For this review, use the dimensioned drawing (mm, ordinates from the lowest corner) and the shaded views. A direction names the side the tool comes from. Give positions to 0.01 mm unless a question says otherwise; leave off trailing zeros. Order: outer loops, then holes, each group sorted by start corner. A loop starts at its lowest first (then second) coordinate and runs counter-clockwise, first axis right, second up. Notation, with made-up numbers: (53, 21) - (62, 21) arc R13 ccw to (62, 37) - close; hole circle Ø4 at (48.25, 59.5). An arc over 180 degrees is marked (long way). Use a Markdown table: item, result. Add a question column.
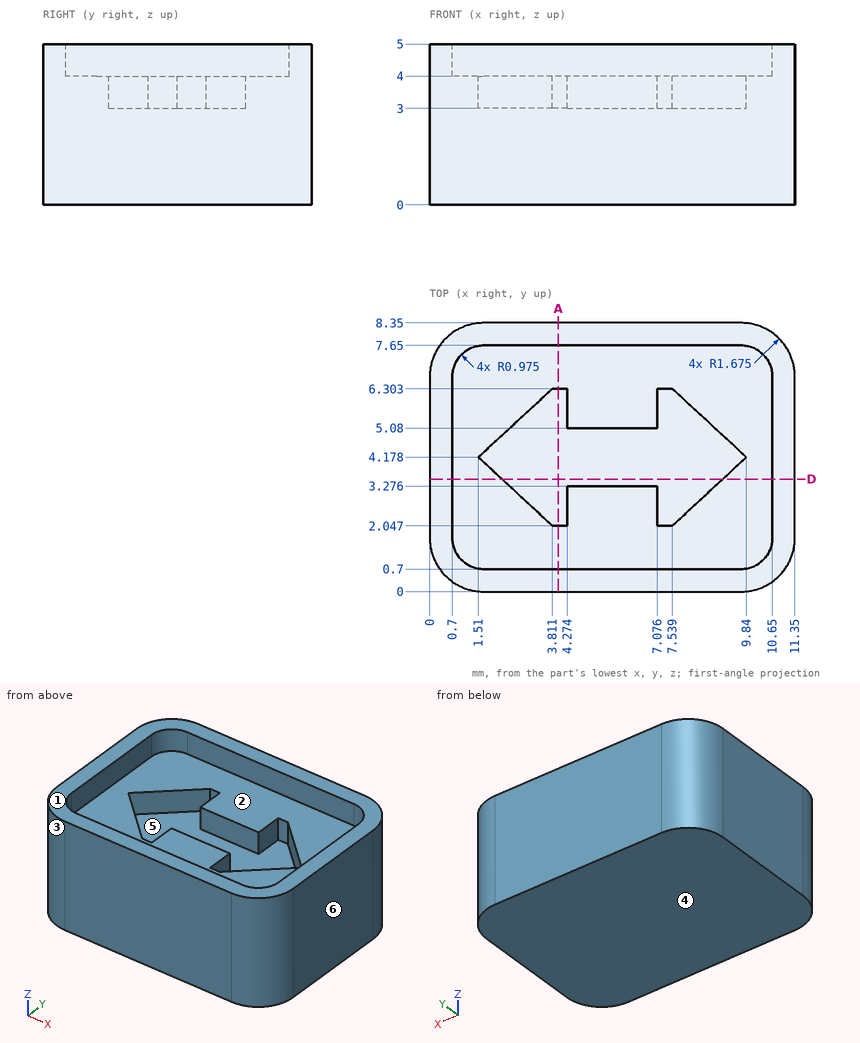
Q1. Clearance check with a flat-ended pin moving along its axis: P1, Ø3.5, axis at x = 7, y = 3.5, coming from the +Z side. State where the tip first meets the part, or that it passes through.
Q2. We need section A-A (x = 4). Write out the cut boundary in (y, z).
Q3. Wall thickness on probe 1 along X at (y, z) = (6.5, 4.3); probe 2 along Z at (x, y) = (6, 2.5); probe 3 along Z at (x, y) = (4.5, 4.25): over which ranges is each line inside the solid? List them lowest first.
Q4. We need section D-D (y = 3.5). Write out the cut boundary in (x, z).
Q5. Machinability: for the marked faces 1 and 2, which of the approach directions +Z, -Z, +X, -X, +Y, -Y give a long, thin tool a straight path to every point of the face, cutting with its end or side? Answer none if there is none.
Q6. Draft analysis for pull direction X (two halves, no side actions). For the marked faces 3, 4, 5 and 6, state which applies: pulls with the +X half, pulls with the -X half, needs draft (parallel to the pull), parting line crosses it, or undercut.
Here are the results:
| question | item | result |
|---|---|---|
| 1 | P1 | z = 4 |
| 2 | outline | (0, 0) - (8.35, 0) - (8.35, 5) - (7.65, 5) - (7.65, 4) - (6.3, 4) - (6.3, 3) - (2.05, 3) - (2.05, 4) - (0.7, 4) - (0.7, 5) - (0, 5) - close |
| 3 | probe 1 | 0 to 0.7, 10.65 to 11.35 |
| 3 | probe 2 | 0 to 4 |
| 3 | probe 3 | 0 to 3 |
| 4 | outline | (0, 0) - (11.35, 0) - (11.35, 5) - (10.65, 5) - (10.65, 4) - (9.11, 4) - (9.11, 3) - (2.24, 3) - (2.24, 4) - (0.7, 4) - (0.7, 5) - (0, 5) - close |
| 5 | face 1 | +Z, +X, -X, +Y, -Y |
| 5 | face 2 | +Z |
| 6 | face 3 | pulls with the -X half |
| 6 | face 4 | needs draft |
| 6 | face 5 | undercut |
| 6 | face 6 | pulls with the +X half |
